Autodesk Inventor part; units mm, degrees
ref_plane "YZ Plane" through (0, 0, 0) normal (1, 0, 0) x (0, 1, 0)
ref_plane "XZ Plane" through (0, 0, 0) normal (0, 1, 0) x (-1, 0, 0)
ref_plane "XY Plane" through (0, 0, 0) normal (0, 0, 1) x (1, 0, 0)
sketch "Sketch1" plane through (0, 0, 0) normal (1, 0, 0) x (0, 1, 0)
  line L0 (50, 10) -> (40, 10)
  line L1 (40, 10) -> (40, -10)
  line L2 (40, -10) -> (50, -10)
  line L3 (50, -10) -> (50, 10)
  line L4 (40, 2.5) -> (0, 2.5)
  line L5 (0, 2.5) -> (0, -2.5)
  line L6 (0, -2.5) -> (40, -2.5)
  line L7 (40, -2.5) -> (40, 2.5)
  point P0 (0, 0)
  dimension "d0" = 40
  dimension "d1" = 10
  dimension "d2" = 5
  dimension "d3" = 2.5
  dimension "d4" = 20
  dimension "d5" = 10
extrude "Extrusion1" add sketch "Sketch1" along normal blind 15
sketch "Sketch2" plane through (15, 0, 0) normal (1, 0, 0) x (0, 0, -1)
  line L0 (-10, 50) -> (-10, 40)
  line L1 (2.5, 40) -> (10, 40)
  line L2 (-10, 50) -> (10, 50)
  line L3 (10, 50) -> (10, 40)
  line L4 (10, 40) -> (-10, 40)
  line L5 (-10, 40) -> (-10, 50)
  point P0 (0, 0)
extrude "Extrusion2" add sketch "Sketch2" along normal blind 10
sketch "Sketch3" plane through (0, 0, 0) normal (-1, 0, 0) x (0, 0, 1)
  line L0 (-10, 40) -> (-10, 50)
  line L1 (10, 50) -> (10, 40)
  line L2 (-10, 50) -> (10, 50)
  line L3 (10, 50) -> (10, 40)
  line L4 (10, 40) -> (-10, 40)
  line L5 (-10, 40) -> (-10, 50)
  point P0 (0, 0)
extrude "Extrusion3" add sketch "Sketch3" along normal blind 10
sketch "Sketch4" plane through (0, 0, -2.5) normal (0, 0, -1) x (-1, 0, 0)
  circle A0 centre (-7.5, 12) radius 6
  point P0 (0, 0)
  dimension "d12" = 12
extrude "Extrusion4" cut sketch "Sketch4" against normal blind 5
sketch "Sketch5" plane through (0, 0, -2.5) normal (0, -1, 0) x (1, 0, 0)
  line L0 (-5, 7.5) -> (20, 7.5)
  line L1 (20, 7.5) -> (20, -2.5)
  line L2 (20, -2.5) -> (-5, -2.5)
  line L3 (-5, -2.5) -> (-5, 7.5)
  point P0 (0, 2.5)
  dimension "d15" = 25
  dimension "d16" = 10
extrude "Extrusion5" add sketch "Sketch5" along normal blind 10
sketch "Sketch6" plane through (20, 0, 5) normal (1, 0, 0) x (0, 0, -1)
  line L0 (0, 0) -> (10, 0)
  arc A0 (0, 0) -> (10, 0) centre (5, 0) ccw
  line L1 (0, 0) -> (0, -10)
  line L2 (0, 0) -> (0, -10)
  line L3 (10, -10) -> (0, -10)
  line L4 (0, -10) -> (10, -10)
  line L5 (10, 0) -> (10, -10)
  line L6 (10, -10) -> (10, 0)
  point P0 (5, 0)
  dimension "d19" = 5
extrude "Extrusion6" cut sketch "Sketch6" against normal blind 25 contours A0 L5 L3 L1
properties part number "Example Follower"
Geometry: final body of the model. Coordinates: model frame, mm. A direction names the side the tool comes from. Round coordinates to 2 decimals unless told otherwise and drop trailing zeros. Loops run counter-clockwise (first coordinate to the right, second up) from the corner with the lowest first, then second, coordinate; pieces in that order, holes last. Notation, with made-up numbers: M 7.5,15.5 L 25.5,15.5 A36 ccw 25.5,49.5 Z; hole C -35.75,7.25 d9. An arc over 180 degrees is marked long. One line per question, with ' | ' between items.
(1) Access query for faces 1 (the flat face through (15, 20, 0)), 2 (the flat face through (-5, -2, 0)), 3 (the flat face through (0, 20, 0)), 4 (the flat face through (8, 40, -4)). Directions: +Z, -Z, +X, -X, +Y, -Y. A direction counts if a zero-diameter tool reaches every point of the face in a straight line with its end or side. Return the directions, or none.
Check result:
face 1: +Z, -Z, +X | face 2: +Z, -Z, -X, -Y | face 3: +Z, -Z, -X | face 4: none
(2) Cut plane C-C on x = 7.5. Return the cut outline in (y, z).
Check result:
outline: M 0,-5 L 0,-2.5 L 6,-2.5 L 6,2.5 L 0,2.5 L 0,5 A5 ccw Z; M 18,-2.5 L 40,-2.5 L 40,-10 L 50,-10 L 50,10 L 40,10 L 40,2.5 L 18,2.5 Z
(3) Pull-direction query (Y, two-part tool) for faces 5 (the flat face through (8, 45, 10)), 6 (the flat face through (7, 20, 2.5)), 7 (the cylindrical face through (8, -5, 0)), 8 (the flat face through (8, 50, 0)); classes: +Y half, -Y half, draft (parallel to the pull), parting line (faces both ways), or undercut.
Check result:
face 5: draft | face 6: undercut | face 7: -Y half | face 8: +Y half
(4) Cut plane A-A on y = 12. Return the cut outline in (x, z).
Check result:
outline: M 0,-2.5 L 1.5,-2.5 L 1.5,2.5 L 0,2.5 Z; M 13.5,-2.5 L 15,-2.5 L 15,2.5 L 13.5,2.5 Z
(5) Cut plane D-D on z = 0. Return the cut outline in (x, y), plus the area to 3 significant figures.
Check result:
outline: M -10,40 L 0,40 L 0,0 L -5,0 L -5,-5 L 20,-5 L 20,0 L 15,0 L 15,40 L 25,40 L 25,50 L -10,50 Z; hole C 7.5,12 d12 | area: 962 mm2
(6) Material intervals for line 1 along X through (y, z) = (32.5, 2); line 2 along Y through (x, z) = (21.5, -0.75); line 3 along X through (y, z) = (8.5, -0.5), sorted ascending. Write a range as from..to.
Check result:
line 1: x = 0..15 | line 2: y = 40..50 | line 3: x = 0..2.63, 12.37..15
(7) Cut plane B-B on z = 4. Return the cut outline in (x, y).
Check result:
outline: M -10,40 L 25,40 L 25,50 L -10,50 Z; M -5,-3 L 20,-3 L 20,0 L -5,0 Z
(8) Contact query for flat-ended pins moving along their axis: P1, Ø8, axis at y = 27, z = 8, coming from the -X side; P2, Ø5, axis at x = 10.5, y = 8, coming from the +Z side; P3, Ø4, axis at y = 20.5, z = -1, coming from the -X side; P4, Ø4, axis at x = -1.5, y = 37, coming from the -Z side. Output: stop coordinate, or through.
Check result:
P1: passes through | P2: stops at z = 2.5 | P3: stops at x = 0 | P4: stops at z = -2.5
